Here's how the part is built. I have some questions about the finished solid (model axes, mm). Face numbers are marked on the shaded views. Give positions to 0.01 mm unless a question says otherwise; leave off trailing zeros. Order: outer loops, then holes, each group sorted by start corner. A loop starts at its lowest first (then second) coordinate and runs counter-clockwise, first axis right, second up. Notation, with made-up numbers: M -37.75,88 L -1.75,88 A18 cw -1.75,113 Z; hole C 33.25,-30 d7. An arc over 180 degrees is marked long. Use one line per item in the form item = value.
from build123d import *

# Parameters (mm, degrees)
F1_DEPTH = 15
F2_W     = 1
F2_H     = 3
F3_DEPTH = 25


with BuildPart() as f1:
    # F0 (on Top) → F1 (new body)
    with BuildSketch(Plane.XY):
        with BuildLine():
            ThreePointArc((-18.455241, 2.525), (-16.669796, 1.785445), (-15.930241, 0))
            Line((-15.930241, 0), (-14.455241, 0))
            ThreePointArc((-14.455241, 0), (-14.639965, 1.201527), (-15.177075, 2.292079))
            ThreePointArc((-15.177075, 2.292079), (-16.607041, 3.547416), (-18.455241, 4))
            Line((-18.455241, 4), (-18.455241, 2.525))
        make_face()
        with BuildLine():
            Line((11.544759, 2.525), (11.544759, 4))
            ThreePointArc((11.544759, 4), (9.69656, 3.547416), (8.266593, 2.292079))
            ThreePointArc((8.266593, 2.292079), (7.729483, 1.201527), (7.544759, 0))
            Line((7.544759, 0), (9.019759, 0))
            ThreePointArc((9.019759, 0), (9.759315, 1.785445), (11.544759, 2.525))
        make_face()
        with BuildLine():
            Line((-14.455241, 0), (-15.930241, 0))
            ThreePointArc((-15.930241, 0), (-20.240685, -1.785445), (-18.455241, 2.525))
            Line((-18.455241, 2.525), (-18.455241, 4))
            ThreePointArc((-18.455241, 4), (-21.283668, -2.828427), (-14.455241, 0))
        make_face()
        with BuildLine():
            ThreePointArc((15.544759, 0), (14.373186, 2.828427), (11.544759, 4))
            Line((11.544759, 4), (11.544759, 2.525))
            ThreePointArc((11.544759, 2.525), (13.330204, 1.785445), (14.069759, 0))
            ThreePointArc((14.069759, 0), (11.544759, -2.525), (9.019759, 0))
            Line((9.019759, 0), (7.544759, 0))
            ThreePointArc((7.544759, 0), (11.544759, -4), (15.544759, 0))
        make_face()
        with BuildLine():
            Line((11.544759, 4), (-18.455241, 4))
            ThreePointArc((-18.455241, 4), (-16.607041, 3.547416), (-15.177075, 2.292079))
            Line((-15.177075, 2.292079), (-12.304623, 2.292079))
            Line((-12.304623, 2.292079), (6.274519, 2.292079))
            Line((6.274519, 2.292079), (8.266593, 2.292079))
            ThreePointArc((8.266593, 2.292079), (9.69656, 3.547416), (11.544759, 4))
        make_face()
    extrude(amount=F1_DEPTH)

    # F2 (on face) → F3 (cut)
    with BuildSketch(Plane.XZ.offset(-2.292079)):
        with Locations((-14.677075, 9)):
            Rectangle(F2_W, F2_H)
        with Locations((7.766593, 9)):
            Rectangle(F2_W, F2_H)
    extrude(amount=-F3_DEPTH, mode=Mode.SUBTRACT)


solid = f1.part
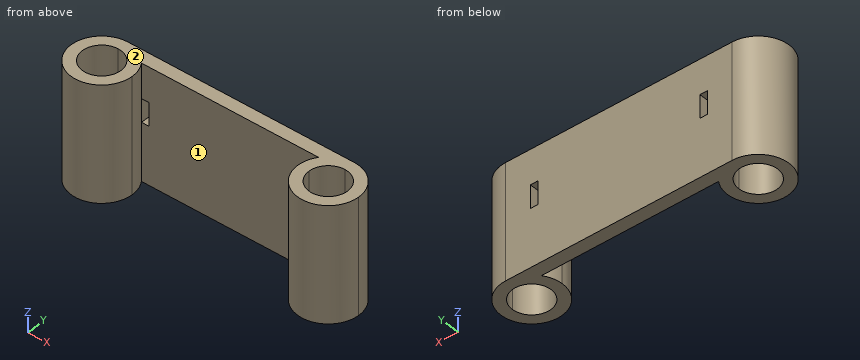
Q1. I'm going to push flat-ended pins straight in: pin 1 Ø0.9 at (y, z) = (3, 9.5) entering from +X; pin 2 Ø0.5 at (y, z) = (3.5, 8.5) entering from -X; pin 3 Ø3 at (x, z) = (9, 4) entering from -Y. Where does each tip first touch, or does it pass through?
Found:
pin_1 = 14.63
pin_2 = -20.79
pin_3 = -3.86
Q2. Thinking about a two-plate mould opening in X: for the marked faces 1 and 2, which applies, +X half, -X half, draft (parallel to the pull), parting line (faces both ways), or undercut?
Found:
face_1 = undercut
face_2 = draft
Q3. I want a section at C-C on x = -17. Write out the boundary of the cut face in (y, z), then the cut area to 3 significant figures.
Found:
outline = M -3.73,0 L -2.06,0 L -2.06,15 L -3.73,15 Z; M 2.06,0 L 4,0 L 4,15 L 2.06,15 Z
area = 54.0 mm²
Q4. I want a section at B-B on z = 6.25. Write out the boundary of the cut face in (x, y) (3 decimals), then the cut area to 3 significant figures.
Found:
outline = M -18.455,4 A4 ccw long -14.455,0 A4 ccw -15.177,2.292 L 8.267,2.292 A4 ccw 7.545,0 A4 ccw long 11.545,4 Z; hole M -18.455,2.525 A2.525 ccw long -15.93,0 A2.525 ccw Z; hole M 11.545,2.525 A2.525 ccw long 14.07,0 A2.525 ccw Z
area = 104 mm²
Q5. I want a section at D-D on x = 0.5. Write out the boundary of the cut face in (y, z).
Found:
outline = M 2.29,0 L 4,0 L 4,15 L 2.29,15 Z
Q6. I want a section at A-A on z = 10. Write out the boundary of the cut face in (x, y) (3 decimals).
Found:
outline = M -18.455,4 A4 ccw long -14.455,0 A4 ccw -15.177,2.292 L -15.177,4 Z; M -14.177,2.292 L 7.267,2.292 L 7.267,4 L -14.177,4 Z; M 7.545,0 A4 ccw long 11.545,4 L 8.267,4 L 8.267,2.292 A4 ccw Z; hole M -18.455,2.525 A2.525 ccw long -15.93,0 A2.525 ccw Z; hole M 11.545,2.525 A2.525 ccw long 14.07,0 A2.525 ccw Z
Q7. I need wall thicknesses on L1, parallel to X at y = -1.75, z = 10.75; L2, parallel to X at y = 2.75, z = 10; L3, parallel to Y at x = -8, z = 0.5. Which ranges of each line are inside material? Lowest first, please.
Found:
L1 = -22.05 to -20.28, -16.64 to -14.86, 7.95 to 9.72, 13.36 to 15.14
L2 = -21.36 to -15.18, -14.18 to 7.27, 8.27 to 14.45
L3 = 2.29 to 4
